The listing builds one solid part. Answer for the finished solid, in the listing's coordinates (mm). A direction names the side the tool comes from. Coordinates: 2 decimals unless noted, no trailing zeros. Order: outer loops, then holes, each group sorted by start corner. A loop starts at its lowest first (then second) coordinate and runs counter-clockwise, first axis right, second up.
from build123d import *

# Parameters (mm, degrees)
F0_R     = 10
F0_R_2   = 0.8
F0_R_3   = 5
F0_R_4   = 1.5
F1_DEPTH = 4
F2_DEPTH = 1


with BuildPart() as f1:
    # F0 (on Top) → F1 (new body)
    with BuildSketch(Plane.XY):
        Circle(F0_R)
        with Locations((-4.949747, -4.949747)):
            Circle(F0_R_2, mode=Mode.SUBTRACT)
        with Locations((0, -7)):
            Circle(F0_R_2, mode=Mode.SUBTRACT)
        with Locations((4.949747, -4.949747)):
            Circle(F0_R_2, mode=Mode.SUBTRACT)
        with Locations((-7, 0)):
            Circle(F0_R_2, mode=Mode.SUBTRACT)
        with Locations((-4.949747, 4.949747)):
            Circle(F0_R_2, mode=Mode.SUBTRACT)
        Circle(F0_R_3, mode=Mode.SUBTRACT)
        with Locations((4.949747, 4.949747)):
            Circle(F0_R_2, mode=Mode.SUBTRACT)
        with Locations((7, 0)):
            Circle(F0_R_2, mode=Mode.SUBTRACT)
        with Locations((0, 7)):
            Circle(F0_R_2, mode=Mode.SUBTRACT)
        Circle(F0_R_3)
        Circle(F0_R_4, mode=Mode.SUBTRACT)
    extrude(amount=-F1_DEPTH)

    # F0 (on Top) → F2 (cut)
    with BuildSketch(Plane.XY):
        Circle(F0_R_3)
        Circle(F0_R_4, mode=Mode.SUBTRACT)
    extrude(amount=-F2_DEPTH, mode=Mode.SUBTRACT)


solid = f1.part
(1) Find section C-C on z = -3.4. Count the separate pieces of the cut face and the enclosed holes in it, then the cut area to 3 significant figures.
(2) Find section A-A on x = 0. Determine the outline of the cut face in (y, z).
(3) The mould has two halves that part along Y. Classify faces 3 (the cylindrical face through (-2.17, -9.76, -1.97)), 4 (the cylindrical face through (4.15, 4.98, -1.97)), 5 (the flat face through (0, -2, -4)): pulls with the +Y half, pulls with the -Y half, needs draft (parallel to the pull), parting line crosses it, or undercut.
(4) Find section B-B on y = 7. Determine the outline of the cut face in (x, z).
(5) Given pin 1 Ø1 at (y, z) = (4.5, -1) entering from +X; pin 2 Ø9 at (x, y) = (0, 0) entering from +Z, each flat-ended and moving along its own axis, determine where each tip first touches the part or whether it passes through.
(6) Find the intervals of material crossed by probe 1 along Y at (x, z) = (0, -2.6); probe 2 along Z at (x, y) = (1, -3.25); probe 3 along X at (y, z) = (-5.5, -2.95), in increasing order.
(7) A tool of negligible diameter and unlimited length cuts with its end or side. For faces 1 (the flat face through (-1.2, 1.2, -1)), 2 (the cylindrical face through (6.2, 0, -2)), from which of +Z, -Z, +X, -X, +Y, -Y can it reach the whole face along a straight path? Write none if from no direction.
Resolved:
1. separate pieces: 1
1. enclosed holes: 9
1. area: 291 mm2
2. outline: (-10, -4) - (-7.8, -4) - (-7.8, 0) - (-10, 0) - close; (-6.2, -4) - (-1.5, -4) - (-1.5, -1) - (-5, -1) - (-5, 0) - (-6.2, 0) - close; (1.5, -4) - (6.2, -4) - (6.2, 0) - (5, 0) - (5, -1) - (1.5, -1) - close; (7.8, -4) - (10, -4) - (10, 0) - (7.8, 0) - close
3. face 3: parting line crosses it
3. face 4: undercut
3. face 5: needs draft
4. outline: (-7.14, -4) - (-0.8, -4) - (-0.8, 0) - (-7.14, 0) - close; (0.8, -4) - (7.14, -4) - (7.14, 0) - (0.8, 0) - close
5. pin 1: stops at x = 9.17
5. pin 2: stops at z = -1
6. probe 1: y = -10 to -7.8, -6.2 to -1.5, 1.5 to 6.2, 7.8 to 10
6. probe 2: z = -4 to -1
6. probe 3: x = -8.35 to -5.53, -4.37 to 4.37, 5.53 to 8.35
7. face 1: +Z
7. face 2: +Z, -Z
